Could you check a few things on this model? Use its own coordinates, in mm. Face numbers are marked on the shaded views. A direction names the side the tool comes from. Give positions to 0.01 mm unless a question says otherwise; leave off trailing zeros. Order: outer loops, then holes, each group sorted by start corner. A loop starts at its lowest first (then second) coordinate and runs counter-clockwise, first axis right, second up. Notation, with made-up numbers: (-28.5, 68.25) - (-15.5, 68.25) arc R19 ccw to (-15.5, 100.25) - close; hole circle Ø6 at (-31, -38.75). An arc over 180 degrees is marked (long way). Put each result on its own line as item: value.
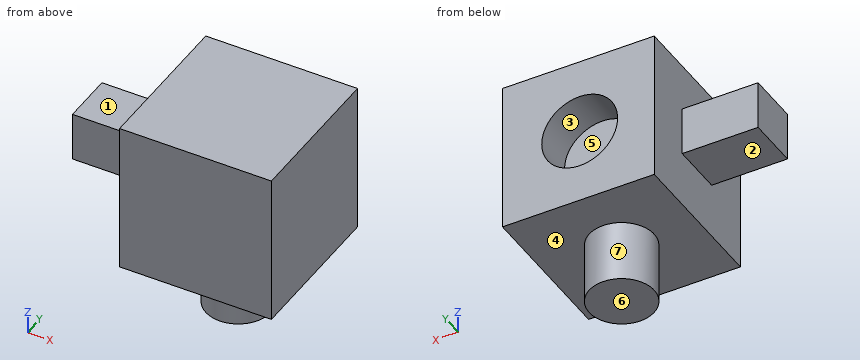
from build123d import *

# Parameters (mm, degrees)
F0_W     = 50.8
F0_H     = 50.8
F1_DEPTH = 50.8
F2_R     = 12.7
F3_DEPTH = 13.462
F4_R     = 10.859331
F5_DEPTH = 20.574
F6_W     = 17.36345
F6_H     = 16.376892
F7_DEPTH = 25.4


with BuildPart() as f1:
    # F0 (on Front) → F1 (new body)
    with BuildSketch(Plane.XZ):
        with Locations((25.4, 25.4)):
            Rectangle(F0_W, F0_H)
    extrude(amount=F1_DEPTH)

    # F2 (on Front) → F3 (cut)
    with BuildSketch(Plane.XZ):
        with Locations((24.959963, 25.354587)):
            Circle(F2_R)
    extrude(amount=F3_DEPTH, mode=Mode.SUBTRACT)

    # F4 (on Top) → F5 (join)
    with BuildSketch(Plane.XY):
        with Locations((24.959963, -24.762653)):
            Circle(F4_R)
    extrude(amount=-F5_DEPTH)

    # F6 (on face) → F7 (join)
    with BuildSketch(Plane(origin=(0, 0, 0), x_dir=(0, -1, 0), z_dir=(-1, 0, 0))):
        with Locations((25.157274, 26.834427)):
            Rectangle(F6_W, F6_H)
    extrude(amount=F7_DEPTH)


solid = f1.part
1) Which directions (+Z, -Z, +X, -X, +Y, -Y) give clear straight access to the entire face, cutting with the end or side of a thin tool? Please do the marked faces 1, 2, 3 and 4.
Filled in:
face 1: +Z, -X, +Y, -Y
face 2: -Z, -X, +Y, -Y
face 3: +Y
face 4: -Z
2) We'd pull the mould along Z, two halves only. Please class the marked faces 5, 6 and 7: pulls with the +Z half, pulls with the -Z half, needs draft (parallel to the pull), parting line crosses it, or undercut.
Filled in:
face 5: undercut
face 6: pulls with the -Z half
face 7: needs draft
3) Suppose I cut it at D-D, the plane y = -12.5. List the corners of the cut face in (x, z) for me, and give its area (3 significant figures).
Filled in:
outline: (0, 0) - (50.8, 0) - (50.8, 50.8) - (0, 50.8) - close; hole circle Ø25.4 at (24.96, 25.35)
area: 2,070 mm^2
4) I'm going to push flat-ended pins straight in: pin 1 (8 mm diameter, centred on y = -30.5, z = -12, fed in from +X); pin 2 (8 mm diameter, centred on x = -17.5, z = 29, fed in from -Y); pin 3 (14 mm diameter, centred on x = -7.5, y = -26.5, fed in from +Z). Where does each tip first touch, or does it pass through?
Filled in:
pin 1: stops at x = 35.68
pin 2: stops at y = -33.84
pin 3: stops at z = 35.02
5) If I drill on line 1 (Z direction, x = -20, y = -27.5); line 2 (Z direction, x = 39, y = -23); line 3 (Z direction, x = 25, y = -12.5), over which ranges is the centre line in solid material (lowest first)? Write a range as [from, to].
Filled in:
line 1: z = [18.65, 35.02]
line 2: z = [0, 50.8]
line 3: z = [0, 12.65], [38.05, 50.8]
6) Suppose I cut it at A-A, the plane y = -27. List the corners of the cut face in (x, z) for me.
Filled in:
outline: (-25.4, 18.65) - (0, 18.65) - (0, 0) - (14.33, 0) - (14.33, -20.57) - (35.59, -20.57) - (35.59, 0) - (50.8, 0) - (50.8, 50.8) - (0, 50.8) - (0, 35.02) - (-25.4, 35.02) - close
7) Suppose I cut it at B-B, the plane x = 32.5. List the corners of the cut face in (y, z) for me, and give its area (3 significant figures).
Filled in:
outline: (-50.8, 0) - (-32.58, 0) - (-32.58, -20.57) - (-16.95, -20.57) - (-16.95, 0) - (0, 0) - (0, 15.14) - (-13.46, 15.14) - (-13.46, 35.57) - (0, 35.57) - (0, 50.8) - (-50.8, 50.8) - close
area: 2,630 mm^2
8) Suppose I cut it at C-C, the plane z = 14. List the corners of the cut face in (x, y) for me.
Filled in:
outline: (0, -50.8) - (50.8, -50.8) - (50.8, 0) - (30.65, 0) - (30.65, -13.46) - (19.27, -13.46) - (19.27, 0) - (0, 0) - close
